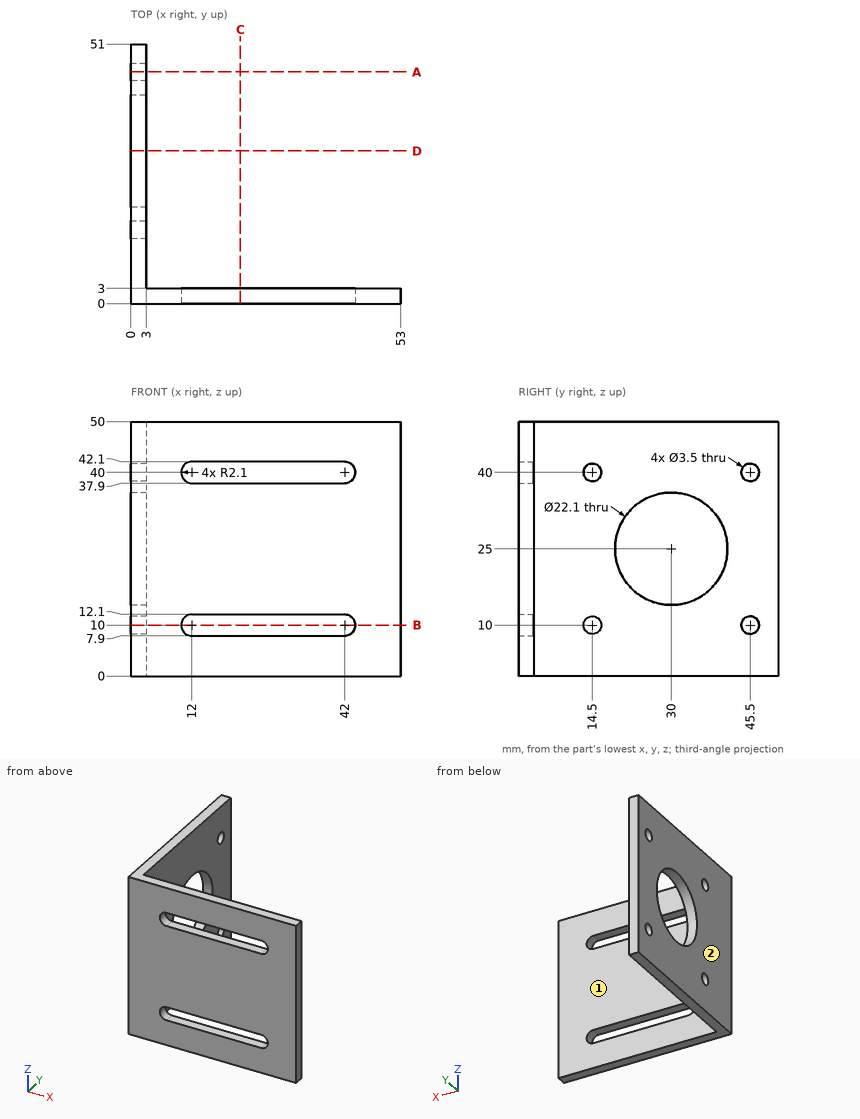
Study the drawing (mm; zero at the part's minimum x, y, z) and answer. A direction names the side the tool comes from. Round coordinates to 2 decimals unless told otherwise and drop trailing zeros. Write each loop counter-clockwise with the first axis right and the second up, starting at its lowest first coordinate (ties: lowest second). Pieces come first, ordered by that corner, then holes. Notation, with made-up numbers: (-35, 85.25) - (-18, 85.25) arc R30 cw to (-18, 107.25) - close; hole circle Ø8 at (32, 46.25). An arc over 180 degrees is marked (long way). Return JSON: item names as keys, results as strings. Group by question number.
Q1. Each of these flat-tipped pins is pushed along its axis until it touches: pin 1 Ø4.5 at (y, z) = (14.5, 40) entering from -X; pin 2 Ø25 at (x, z) = (16, 19.5) entering from +Y; pin 3 Ø4 at (y, z) = (45.5, 40) entering from +X; pin 4 Ø20 at (y, z) = (30, 25) entering from +X. Where does it stop, or does it pass through?
Q2. The part is cut by section C-C on x = 21.5. Write down the section's boundary in (y, z).
Q3. The part is cut by section D-D on y = 30. Write down the section's boundary in (x, z).
Q4. For the marked faces 1 and 2, determine the directions among +Z, -Z, +X, -X, +Y, -Y from which every point of the face is accessible in a straight line to the end or side of a thin tool.
Q5. The part is cut by section A-A on y = 45.5. Write down the section's boundary in (x, z), then the cut area to 3 significant figures.
Q6. Find the intervals of material crossed by L1, parallel to Z at x = 1.6, y = 14.5; L2, parallel to Y at x = 1, z = 10; L3, parallel to Y at x = 1.05, z = 25, in increasing order.
Q7. The part is cut by section B-B on z = 10. Write down the section's boundary in (x, y).
Solved:
{
 "1": {"pin 1": "x = 0", "pin 2": "y = 3", "pin 3": "x = 3", "pin 4": "through"},
 "2": {"outline": "(0, 0) - (3, 0) - (3, 7.9) - (0, 7.9) - close; (0, 12.1) - (3, 12.1) - (3, 37.9) - (0, 37.9) - close; (0, 42.1) - (3, 42.1) - (3, 50) - (0, 50) - close"},
 "3": {"outline": "(0, 0) - (3, 0) - (3, 13.95) - (0, 13.95) - close; (0, 36.05) - (3, 36.05) - (3, 50) - (0, 50) - close"},
 "4": {"face 1": "+Z, -Z, +X, +Y", "face 2": "+Z, -Z, -X, +Y, -Y"},
 "5": {"outline": "(0, 0) - (3, 0) - (3, 8.25) - (0, 8.25) - close; (0, 11.75) - (3, 11.75) - (3, 38.25) - (0, 38.25) - close; (0, 41.75) - (3, 41.75) - (3, 50) - (0, 50) - close", "area": "129 mm²"},
 "6": {"L1": "0 to 8.25, 11.75 to 38.25, 41.75 to 50", "L2": "0 to 12.75, 16.25 to 43.75, 47.25 to 51", "L3": "0 to 18.95, 41.05 to 51"},
 "7": {"outline": "(0, 0) - (9.9, 0) - (9.9, 3) - (3, 3) - (3, 12.75) - (0, 12.75) - close; (0, 16.25) - (3, 16.25) - (3, 43.75) - (0, 43.75) - close; (0, 47.25) - (3, 47.25) - (3, 51) - (0, 51) - close; (44.1, 0) - (53, 0) - (53, 3) - (44.1, 3) - close"}
}
